Check sheet for the modelled part. Datum: model origin and axes. Units: mm. Coordinates: 2 decimals unless noted, no trailing zeros. Order: outer loops, then holes, each group sorted by start corner. A loop starts at its lowest first (then second) coordinate and runs counter-clockwise, first axis right, second up.
1. Thickness scan on line 1 (X direction, y = 0.55, z = -2.25); line 2 (Z direction, x = 100, y = 1.45). Record the ranges inside material, lowest first.
2. Gauge pin test, flat end, axial feed: pin 1 Ø4 at (x, z) = (100, 0) entering from +Y. Record the tip position at first contact, or that the pin passes through.
3. Cross-section at B-B (z = 0). Enter the section's corners in (x, y), then the cut area to 3 significant figures.
4. Cross-section at A-A (x = 100). Enter the section's corners in (y, z).
```python
from build123d import *

# Parameters (mm, degrees)
SKETCH1_W                 = 220
SKETCH1_H                 = 12
BOSS_EXTRUDE1_DEPTH       = 2
F_5_0MM_DOWEL_HOLE1_D     = 5
F_5_0MM_DOWEL_HOLE1_DEPTH = 2


with BuildPart() as part:
    # Sketch1 → Boss-Extrude1 (new body)
    with BuildSketch(Plane(origin=(0, 0, 0), x_dir=(1, 0, 0), z_dir=(0, 1, 0))):
        Rectangle(SKETCH1_W, SKETCH1_H)
    extrude(amount=BOSS_EXTRUDE1_DEPTH)

    # Ø5.0mm Dowel Hole1
    with Locations(Plane(origin=(0, 2, 0), x_dir=(1, 0, 0), z_dir=(0, 1, 0))):
        with Locations((-100, 0), (100, 0)):
            Hole(F_5_0MM_DOWEL_HOLE1_D / 2, depth=F_5_0MM_DOWEL_HOLE1_DEPTH)


solid = part.part
```
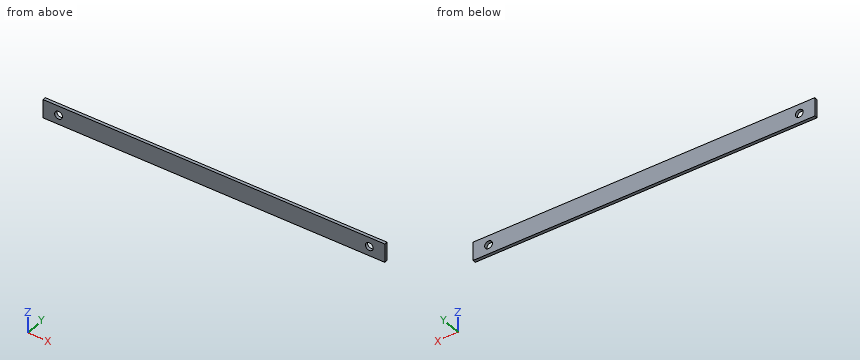
Data:
1. line 1: x = -110 to -101.09, -98.91 to 98.91, 101.09 to 110
1. line 2: z = -6 to -2.5, 2.5 to 6
2. pin 1: passes through
3. outline: (-110, 0) - (-102.5, 0) - (-102.5, 2) - (-110, 2) - close; (-97.5, 0) - (97.5, 0) - (97.5, 2) - (-97.5, 2) - close; (102.5, 0) - (110, 0) - (110, 2) - (102.5, 2) - close
3. area: 420 mm2
4. outline: (0, -6) - (2, -6) - (2, -2.5) - (0, -2.5) - close; (0, 2.5) - (2, 2.5) - (2, 6) - (0, 6) - close
